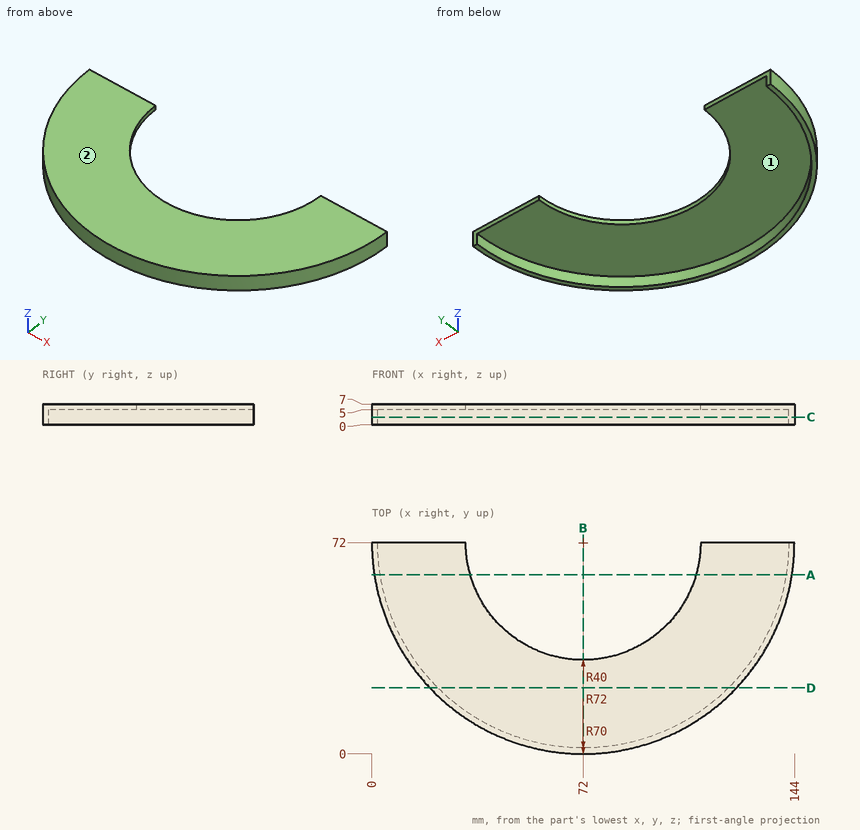
The figure shows three views and two pictorial views of one solid part (mm, origin at its lowest corner). Answer the questions. Round coordinates to 2 decimals unless told otherwise and drop trailing zeros. Order: outer loops, then holes, each group sorted by start corner. A loop starts at its lowest first (then second) coordinate and runs counter-clockwise, first axis right, second up. Notation, with made-up numbers: (28.5, 26.5) - (52.5, 26.5) arc R26 ccw to (52.5, 58.5) - close; hole circle Ø5 at (-16.75, -31). An arc over 180 degrees is marked (long way). Write item = value, one per line. Start each with the question number.
1) For a pull along X with two mould halves and no side action, classify the marked faces 1 and 2 as released by +X, released by -X, zero draft, split by the parting line, or undercut.
2) Given pin 1 (1.5 mm diameter, centred on x = 57.5, z = 1, fed in from +Y); pin 2 (1.5 mm diameter, centred on x = 47.5, z = 1.5, fed in from -Y); pin 3 (2 mm diameter, centred on y = 58, z = 1.5, fed in from +X), each flat-ended and moving along its own axis, determine where each tip first touches the part or whether it passes through.
3) Section D-D, the plane y = 22.5 is taken. Write down the section's boundary in (x, z).
4) Section A-A, the plane y = 61 is taken. Write down the section's boundary in (x, z).
5) Section C-C, the plane z = 2.5 is taken. Write down the section's boundary in (x, y), plus the area to 3 significant figures.
6) Straight lines are drawn through the part: L1, parallel to X at y = 7, z = 4.5; L2, parallel to X at y = 69.5, z = 6; L3, parallel to Z at x = 35.5, y = 17. For each, find the intervals that lie inside material, in ascending order.
7) Section B-B, the plane x = 72 is taken. Write down the section's boundary in (y, z), plus the area to 3 significant figures.
Results list:
q1.face_1 = undercut
q1.face_2 = zero draft
q2.pin_1 = 3.68
q2.pin_2 = 4.03
q2.pin_3 = 142.82
q3.outline = (19.71, 0) - (22.51, 0) - (22.51, 5) - (121.49, 5) - (121.49, 0) - (124.29, 0) - (124.29, 7) - (19.71, 7) - close
q4.outline = (0.85, 0) - (2.87, 0) - (2.87, 5) - (33.54, 5) - (33.54, 7) - (0.85, 7) - close; (110.46, 5) - (141.13, 5) - (141.13, 0) - (143.15, 0) - (143.15, 7) - (110.46, 7) - close
q5.outline = (0, 72) arc R72 ccw to (144, 72) - (142, 72) arc R70 cw to (2, 72) - close
q5.area = 446 mm^2
q6.L1 = 41.03 to 46.02, 97.98 to 102.97
q6.L2 = 0.04 to 32.08, 111.92 to 143.96
q6.L3 = 5 to 7
q7.outline = (0, 0) - (2, 0) - (2, 5) - (32, 5) - (32, 7) - (0, 7) - close
q7.area = 74.0 mm^2
